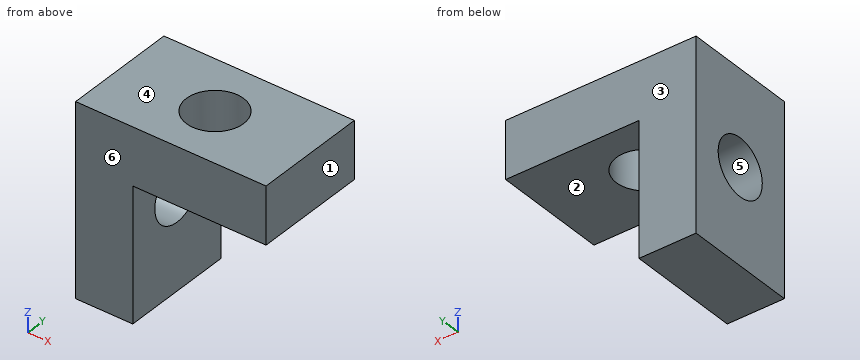
```python
from build123d import *

# Parameters (mm, degrees)
EXTRUDE_1_DEPTH     = 6
SKETCH_2_R          = 1.5
CUT_EXTRUDE_1_DEPTH = 6
SKETCH_3_R          = 1.5
CUT_EXTRUDE_2_DEPTH = 6


with BuildPart() as part:
    # 草图1 → 凸台-拉伸1 (new body)
    with BuildSketch(Plane(origin=(0, 0, 0), x_dir=(1, 0, 0), z_dir=(0, 1, 0))):
        Polygon((0, 0), (10, 0), (10, 3), (3, 3), (3, 10), (0, 10), align=None)
    extrude(amount=EXTRUDE_1_DEPTH)

    # 草图2 → 切除-拉伸1 (cut)
    with BuildSketch(Plane.XY):
        with Locations((5, 3)):
            Circle(SKETCH_2_R)
    extrude(amount=-CUT_EXTRUDE_1_DEPTH, mode=Mode.SUBTRACT)

    # 草图3 → 切除-拉伸2 (cut)
    with BuildSketch(Plane.ZY):
        with Locations((-5, 3)):
            Circle(SKETCH_3_R)
    extrude(amount=-CUT_EXTRUDE_2_DEPTH, mode=Mode.SUBTRACT)


solid = part.part
```
The listing builds one solid part. Answer for the finished solid, in the listing's coordinates (mm). Face numbers are marked on the shaded views. A direction names the side the tool comes from. Round coordinates to 2 decimals unless told otherwise and drop trailing zeros. Loops run counter-clockwise (first coordinate to the right, second up) from the corner with the lowest first, then second, coordinate; pieces in that order, holes last.
1) Given P1, Ø1.5, axis at x = 5, z = -1.5, coming from the -Y side; P2, Ø3, axis at y = 4, z = -9, coming from the +X side, each flat-ended and moving along its own axis, determine where each tip first touches the part or whether it passes through.
Outcome:
P1: stops at y = 0
P2: stops at x = 3
2) For the marked faces 1 and 2, determine the directions among +Z, -Z, +X, -X, +Y, -Y from which every point of the face is accessible in a straight line to the end or side of a thin tool.
Outcome:
face 1: +Z, -Z, +X, +Y, -Y
face 2: -Z, +X, +Y, -Y
3) A cutting plane is placed at A-A on z = -5. Determine the outline of the cut face in (x, y), plus the area to 3 significant figures.
Outcome:
outline: (0, 0) - (3, 0) - (3, 1.5) - (0, 1.5) - close; (0, 4.5) - (3, 4.5) - (3, 6) - (0, 6) - close
area: 9.00 mm2
4) For a pull along Y with two mould halves and no side action, classify the marked faces 3, 4, 5 and 6 as released by +Y, released by -Y, zero draft, split by the parting line, or undercut.
Outcome:
face 3: released by +Y
face 4: zero draft
face 5: undercut
face 6: released by -Y
5) Consider line 1 (Y direction, x = 1.7, z = -5); line 2 (Z direction, x = 7.5, y = 1.6); line 3 (X direction, y = 0.9, z = -3.75). Determine where each line is inside the solid, lowest interval first.
Outcome:
line 1: y = 0 to 1.5, 4.5 to 6
line 2: z = -3 to 0
line 3: x = 0 to 3
6) A cutting plane is placed at D-D on x = 2. Determine the outline of the cut face in (y, z).
Outcome:
outline: (0, -10) - (6, -10) - (6, 0) - (0, 0) - close; hole circle Ø3 at (3, -5)
7) A cutting plane is placed at C-C on x = 5. Determine the outline of the cut face in (y, z), plus the area to 3 significant figures.
Outcome:
outline: (0, -3) - (1.5, -3) - (1.5, 0) - (0, 0) - close; (4.5, -3) - (6, -3) - (6, 0) - (4.5, 0) - close
area: 9.00 mm2
8) A cutting plane is placed at B-B on y = 3. Determine the outline of the cut face in (x, z), plus the area to 3 significant figures.
Outcome:
outline: (0, -10) - (3, -10) - (3, -6.5) - (0, -6.5) - close; (0, -3.5) - (3, -3.5) - (3, -3) - (3.5, -3) - (3.5, 0) - (0, 0) - close; (6.5, -3) - (10, -3) - (10, 0) - (6.5, 0) - close
area: 33.0 mm2
